from build123d import *

# Parameters (mm, degrees)
F1_DEPTH = 12.5
F2_R     = 15
F3_DEPTH = 5.9234467243


with BuildPart() as f1:
    # F0 (on Right) → F1 (new body, symmetric)
    with BuildSketch(Plane.YZ):
        Polygon((23.5929106708, 0), (23.5929106708, 39.6152098016), (51.0941416978, 65), (44.3114793878, 72.3481624906), (18.5929106708, 48.6088444054), (7.9668510469, 66.0182343106), (27.3548236127, 90.718568717), (23.2852262267, 95.1274662114), (0, 65.4620191113), (13.5929106708, 43.1918371068), (13.5929106708, 0), align=None)
    extrude(amount=F1_DEPTH, both=True)

    # F2 (on face) → F3 (cut, through all)
    with BuildSketch(Plane(origin=(0, -31.7941860417, 24.9561320338), x_dir=(1, 0, 0), z_dir=(0, -0.7866188975, 0.6174388311))):
        with Locations((-20.5, 67.0375549689)):
            Circle(F2_R)
        with BuildLine():
            ThreePointArc((35.5, 67.0375549689), (20.5, 82.0375549689), (5.5, 67.0375549689))
            ThreePointArc((5.5, 67.0375549689), (20.5, 52.0375549689), (35.5, 67.0375549689))
        make_face()
        with BuildLine():
            ThreePointArc((-12.5, 79.7261325093), (-7.3660744634, 74.283243342), (-5.5, 67.0375549689))
            Line((-5.5, 67.0375549689), (-5.5, 89.206265453))
            Line((-5.5, 89.206265453), (-12.5, 89.206265453))
            Line((-12.5, 89.206265453), (-12.5, 79.7261325093))
        make_face()
        with BuildLine():
            Line((12.5, 89.206265453), (5.5, 89.206265453))
            Line((5.5, 89.206265453), (5.5, 67.0375549689))
            ThreePointArc((5.5, 67.0375549689), (7.3660744634, 74.283243342), (12.5, 79.7261325093))
            Line((12.5, 79.7261325094), (12.5, 89.206265453))
        make_face()
    extrude(amount=-F3_DEPTH, mode=Mode.SUBTRACT)


solid = f1.part
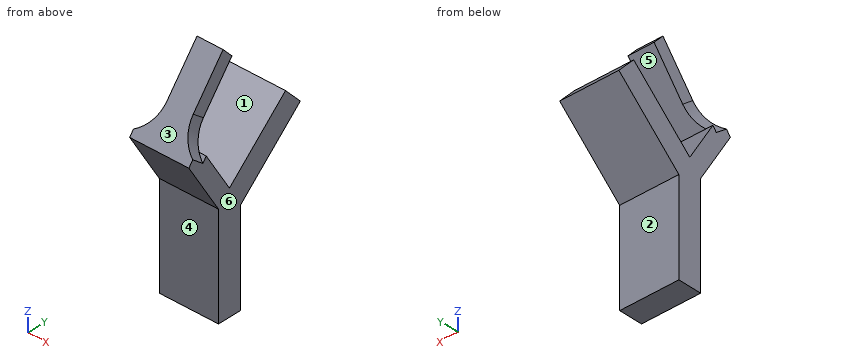
Read the model definition and answer for the solid it produces. Units are mm, in the model's axes. Face numbers are marked on the shaded views. A direction names the side the tool comes from. Coordinates: 2 decimals unless noted, no trailing zeros. Loops run counter-clockwise (first coordinate to the right, second up) from the corner with the lowest first, then second, coordinate; pieces in that order, holes last. Notation, with made-up numbers: (88.25, -6) - (120.25, -6) arc R21 cw to (120.25, 8) - close; hole circle Ø7 at (38.25, 71.5). An arc over 180 degrees is marked (long way). Answer in a Markdown table with one row per item.
Q1. Find section A-A on x = 1. Write down the section's boundary in (y, z).
Here are the results:
| item | result |
|---|---|
| outline | (0, 65.46) - (13.59, 43.19) - (13.59, 0) - (23.59, 0) - (23.59, 39.62) - (51.09, 65) - (44.31, 72.35) - (18.59, 48.61) - (7.97, 66.02) - (27.35, 90.72) - (23.29, 95.13) - close |
Q2. Given P1, Ø6, axis at x = -4.5, z = 67.5, coming from the +Y side; P2, Ø12, axis at x = -6.5, z = 80.5, coming from the +Y side; P3, Ø14, axis at y = 19.5, z = 89, coming from the +X side, each flat-ended and moving along its own axis, determine where each tip first touches the part or whether it passes through.
Here are the results:
| item | result |
|---|---|
| P1 | stops at y = 51.09 |
| P2 | stops at y = 23.98 |
| P3 | stops at x = 5.5 |
Q3. For the marked faces 1, 2 and 3, determine the directions among +Z, -Z, +X, -X, +Y, -Y from which every point of the face is accessible in a straight line to the end or side of a thin tool.
Here are the results:
| item | result |
|---|---|
| face 1 | +X, -X |
| face 2 | -Z, +X, -X, +Y |
| face 3 | +Z, +X, -X, -Y |
Q4. Find section D-D on z = 28. Write down the section's boundary in (x, y), plus the area to 3 significant figures.
Here are the results:
| item | result |
|---|---|
| outline | (-12.5, 13.59) - (12.5, 13.59) - (12.5, 23.59) - (-12.5, 23.59) - close |
| area | 250 mm^2 |
Q5. Straight lines are drawn through the part: line 1 along Y through (x, z) = (-1.75, 21); line 2 along Z through (x, y) = (4.25, 20.5); line 3 along Y through (x, z) = (6, 61). For each, find the intervals that lie inside material, in ascending order. Write a range as [from, to].
Here are the results:
| item | result |
|---|---|
| line 1 | y = [13.59, 23.59] |
| line 2 | z = [0, 50.37], [81.99, 91.58] |
| line 3 | y = [2.72, 11.03], [32.02, 46.76] |
Q6. The mould has two halves that part along Y. Classify the marked faces 4, 5 and 6: pulls with the +Y half, pulls with the -Y half, needs draft (parallel to the pull), parting line crosses it, or undercut.
Here are the results:
| item | result |
|---|---|
| face 4 | pulls with the -Y half |
| face 5 | undercut |
| face 6 | needs draft |
Q7. Find section B-B on z = 54.5. Write down the section's boundary in (x, y), plus the area to 3 significant figures.
Here are the results:
| item | result |
|---|---|
| outline | (-12.5, 6.69) - (12.5, 6.69) - (12.5, 15) - (-12.5, 15) - close; (-12.5, 24.98) - (12.5, 24.98) - (12.5, 39.72) - (-12.5, 39.72) - close |
| area | 576 mm^2 |
Q8. Find section C-C on y = 17. Write down the section's boundary in (x, z), plus the area to 3 significant figures.
Here are the results:
| item | result |
|---|---|
| outline | (-12.5, 0) - (12.5, 0) - (12.5, 51.22) - (-12.5, 51.22) - close; (-5.5, 77.53) - (5.5, 77.53) - (5.5, 87.12) - (-5.5, 87.12) - close |
| area | 1,390 mm^2 |
